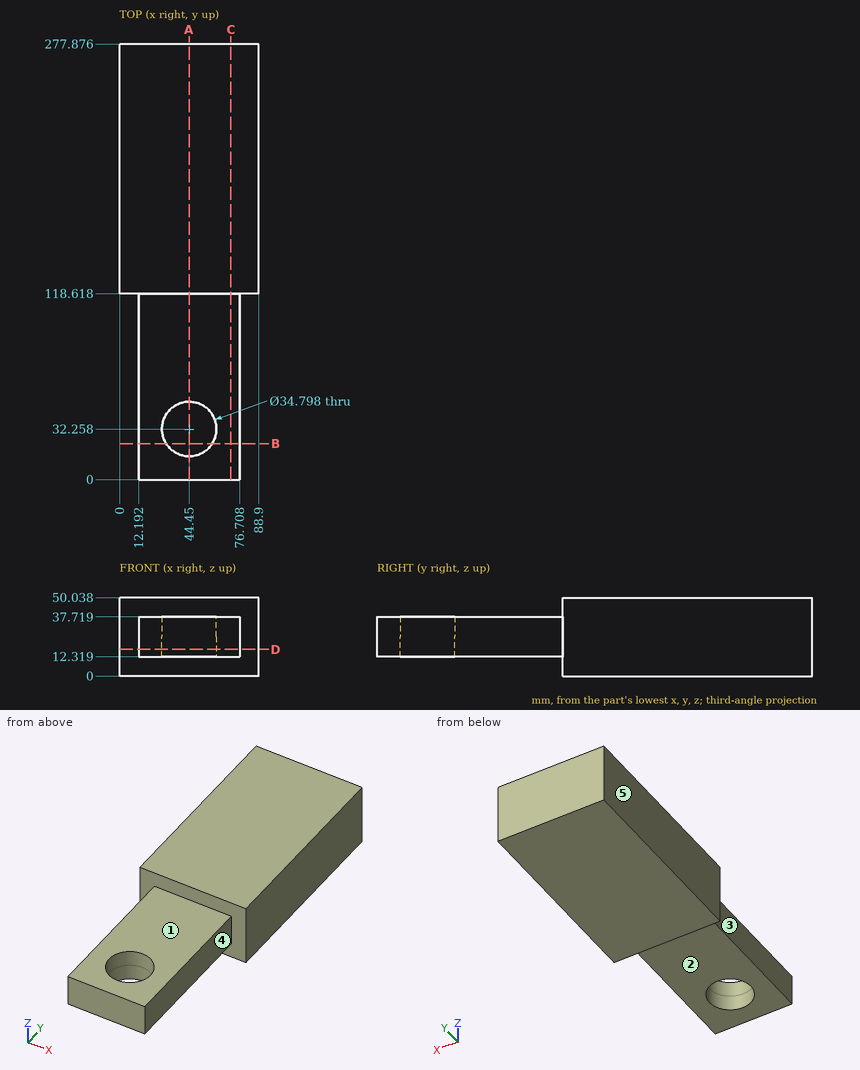
Study the drawing (mm; zero at the part's minimum x, y, z) and answer. A direction names the side the tool comes from. Round coordinates to 2 decimals unless told otherwise and drop trailing zeros. Write each loop counter-clockwise with the first axis right and the second up, starting at its lowest first coordinate (ties: lowest second). Pieces come first, ordered by that corner, then holes.
1) Consider probe 1 along Y at (x, z) = (45.5, 15); probe 2 along Y at (x, z) = (44.45, 32.25); probe 3 along X at (y, z) = (36.5, 31.5). Determine where each line is inside the solid, lowest interval first.
2) A cutting plane is placed at B-B on y = 23. Determine the outline of the cut face in (x, z), and give its area (3 significant figures).
3) Which of the six approach directions +Z, -Z, +X, -X, +Y, -Y give full straight-line access (tool end or side, diameter ignored) to the marked faces 1, 2, 3, 4 and 5?
4) Flat-ended cylindrical pins translate along their axes: P1, Ø1, axis at x = 40, y = 187.5, coming from the -Z side; P2, Ø4, axis at y = 46, z = 40, coming from the -X side; P3, Ø1.5, axis at x = 39.5, z = 10, coming from the -Y side; P4, Ø7.5, axis at y = 31.5, z = 30.5, coming from the +X side. Find the tip coordinate at first contact, or state that the pin passes through.
5) A cutting plane is placed at C-C on x = 71. Determine the outline of the cut face in (y, z).
6) A cutting plane is placed at D-D on z = 17. Determine the outline of the cut face in (x, y).
7) A cutting plane is placed at A-A on x = 44.45. Determine the outline of the cut face in (y, z).
Entries:
1. probe 1: y = 0 to 14.89, 49.63 to 277.88
1. probe 2: y = 0 to 14.86, 49.66 to 277.88
1. probe 3: x = 12.19 to 27.58, 61.32 to 76.71
2. outline: (12.19, 12.32) - (29.72, 12.32) - (29.72, 37.72) - (12.19, 37.72) - close; (59.18, 12.32) - (76.71, 12.32) - (76.71, 37.72) - (59.18, 37.72) - close
2. area: 890 mm2
3. face 1: +Z, +X, -X, -Y
3. face 2: -Z, +X, -X, -Y
3. face 3: +Z, -Z, -X, -Y
3. face 4: +Z, -Z, +X, -Y
3. face 5: +Z, -Z, -X, +Y, -Y
4. P1: stops at z = 0
4. P2: passes through
4. P3: stops at y = 118.62
4. P4: stops at x = 76.71
5. outline: (0, 12.32) - (118.62, 12.32) - (118.62, 0) - (277.88, 0) - (277.88, 50.04) - (118.62, 50.04) - (118.62, 37.72) - (0, 37.72) - close
6. outline: (0, 118.62) - (12.19, 118.62) - (12.19, 0) - (76.71, 0) - (76.71, 118.62) - (88.9, 118.62) - (88.9, 277.88) - (0, 277.88) - close; hole circle Ø34.8 at (44.45, 32.26)
7. outline: (0, 12.32) - (14.86, 12.32) - (14.86, 37.72) - (0, 37.72) - close; (49.66, 12.32) - (118.62, 12.32) - (118.62, 0) - (277.88, 0) - (277.88, 50.04) - (118.62, 50.04) - (118.62, 37.72) - (49.66, 37.72) - close
